```python
from build123d import *

# Parameters (mm, degrees)
SKETCH_R  = 2.2
PAD_DEPTH = 2


with BuildPart() as part:
    # Sketch → Pad (new body)
    with BuildSketch(Plane.XY):
        with BuildLine():
            ThreePointArc((12, -6.2), (16.384062, -4.384062), (18.2, 0))
            Line((18.2, 0), (18.2, 50))
            Line((18.2, 50), (0, 50))
            Line((0, -6.2), (0, 50))
            Line((12, -6.2), (0, -6.2))
        make_face()
        with Locations((12, 0)):
            Circle(SKETCH_R, mode=Mode.SUBTRACT)
        with BuildLine():
            ThreePointArc((12, 6.2), (7.615938, 4.384062), (5.8, 0))
            Line((5.8, 0), (5.8, -2.2))
            Line((5.8, -2.2), (2, -2.2))
            Line((2, 46), (2, -2.2))
            Line((14.2, 46), (2, 46))
            Line((14.2, 46), (14.2, 6.2))
            Line((12, 6.2), (14.2, 6.2))
        make_face(mode=Mode.SUBTRACT)
    pad = extrude(amount=PAD_DEPTH)

    # Mirrored: Pad across Sketch V_Axis
    add(pad.mirror(Plane(origin=(0, 0, 0), x_dir=(0, 0, 1), z_dir=(1, 0, 0))))


solid = part.part
```
Check sheet for the modelled part. Datum: model origin and axes. Units: mm. A direction names the side the tool comes from. Coordinates: 2 decimals unless noted, no trailing zeros. Loops run counter-clockwise (first coordinate to the right, second up) from the corner with the lowest first, then second, coordinate; pieces in that order, holes last.
1) Gauge pin test, flat ends, axial feed: pin 1 (0.6 mm diameter, centred on y = -1, z = 0.5, fed in from +X); pin 2 (3.5 mm diameter, centred on x = 12, y = 0, fed in from -Z). Record the tip position at first contact, or that the pin passes through.
2) Sectioned sample at A-A (x = 5). Record the boundary of the cut face in (y, z), and give its area (3 significant figures).
3) Sectioned sample at B-B (y = 40). Record the boundary of the cut face in (x, z), and give its area (3 significant figures).
4) Release check for a two-part mould opening along Y. For faces 1 (the face through (0, -6.2, 1)), 2 (the face through (-14.032, -0.843, 0.986)), 3 (the face through (0, 22, 2)) record: released by +Y, released by -Y, zero draft, split by the parting line, or undercut.
5) Material ranges on probe 1 along X at (y, z) = (42.5, 0.6); probe 2 along Y at (x, z) = (12, 0.5); probe 3 along Y at (x, z) = (-3.5, 0.6), recorded low to high.
6) Sectioned sample at D-D (x = 13). Record the boundary of the cut face in (y, z).
7) Access from +Z, -Z, +X, -X, +Y, -Y to the whole of each face (thin tool, end or side, straight path). Record for faces 4 (the face through (18.2, 25, 1)), 5 (the face through (2, 22, 1)).
8) Sectioned sample at C-C (z = 0.4). Record the boundary of the cut face in (x, y).
Check sheet entries:
1. pin 1: stops at x = 18.16
1. pin 2: passes through
2. outline: (-6.2, 0) - (-2.2, 0) - (-2.2, 2) - (-6.2, 2) - close; (46, 0) - (50, 0) - (50, 2) - (46, 2) - close
2. area: 16.0 mm2
3. outline: (-18.2, 0) - (-14.2, 0) - (-14.2, 2) - (-18.2, 2) - close; (-2, 0) - (2, 0) - (2, 2) - (-2, 2) - close; (14.2, 0) - (18.2, 0) - (18.2, 2) - (14.2, 2) - close
3. area: 24.0 mm2
4. face 1: released by -Y
4. face 2: undercut
4. face 3: zero draft
5. probe 1: x = -18.2 to -14.2, -2 to 2, 14.2 to 18.2
5. probe 2: y = -6.2 to -2.2, 2.2 to 6.2, 46 to 50
5. probe 3: y = -6.2 to -2.2, 46 to 50
6. outline: (-6.12, 0) - (-1.96, 0) - (-1.96, 2) - (-6.12, 2) - close; (1.96, 0) - (6.2, 0) - (6.2, 2) - (1.96, 2) - close; (46, 0) - (50, 0) - (50, 2) - (46, 2) - close
7. face 4: +Z, -Z, +X, +Y, -Y
7. face 5: +Z, -Z
8. outline: (-18.2, 0) arc R6.2 ccw to (-12, -6.2) - (12, -6.2) arc R6.2 ccw to (18.2, 0) - (18.2, 50) - (-18.2, 50) - close; hole circle Ø4.4 at (-12, 0); hole (-14.2, 6.2) - (-12, 6.2) arc R6.2 cw to (-5.8, 0) - (-5.8, -2.2) - (-2, -2.2) - (-2, 46) - (-14.2, 46) - close; hole (2, -2.2) - (5.8, -2.2) - (5.8, 0) arc R6.2 cw to (12, 6.2) - (14.2, 6.2) - (14.2, 46) - (2, 46) - close; hole circle Ø4.4 at (12, 0)
